Input: dimensioned drawing with shaded views. Units: mm. Origin: part minimum x, y, z. Coordinates: 2 decimals unless noted, no trailing zeros. Order: outer loops, then holes, each group sorted by start corner. A loop starts at its lowest first (then second) coordinate and runs counter-clockwise, first axis right, second up. Notation, with made-up numbers: (-13.75, 37.25) -> (-1.75, 37.25) arc R20 cw to (-1.75, 67.25) -> close; hole circle Ø9 at (-35, 73.5). An arc over 180 degrees is marked (long way). Answer as CSV lines item,"result".
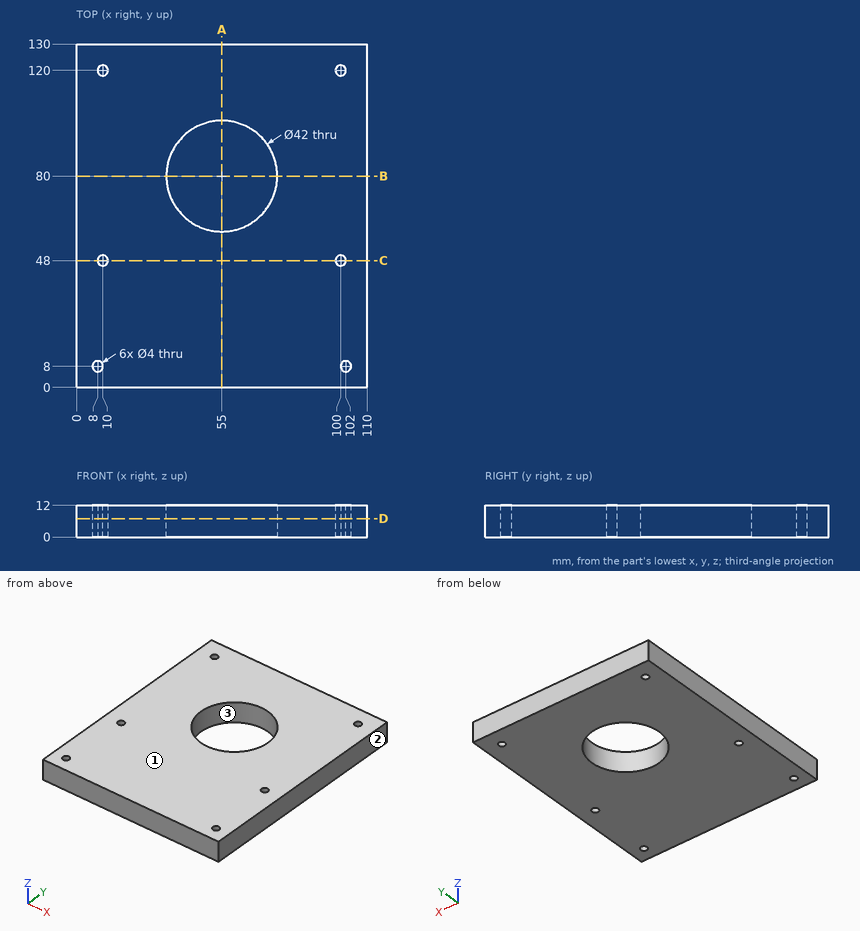
1. Contact query for flat-ended pins moving along their axis: pin 1 (5 mm diameter, centred on y = 20, z = 5.5, fed in from -X); pin 2 (3 mm diameter, centred on x = 102, y = 8, fed in from +Z). Output: stop coordinate, or through.
Findings:
pin 1,"stops at x = 0"
pin 2,"passes through"
2. Cut plane C-C (y = 48). Return the cut outline in (x, z), plus the area to 3 significant figures.
Findings:
outline,"(0, 0) -> (8, 0) -> (8, 12) -> (0, 12) -> close; (12, 0) -> (98, 0) -> (98, 12) -> (12, 12) -> close; (102, 0) -> (110, 0) -> (110, 12) -> (102, 12) -> close"
area,"1,220 mm2"
3. Cut plane A-A (x = 55). Return the cut outline in (y, z), plus the area to 3 significant figures.
Findings:
outline,"(0, 0) -> (59, 0) -> (59, 12) -> (0, 12) -> close; (101, 0) -> (130, 0) -> (130, 12) -> (101, 12) -> close"
area,"1,060 mm2"
4. Cut plane D-D (z = 7). Return the cut outline in (x, y).
Findings:
outline,"(0, 0) -> (110, 0) -> (110, 130) -> (0, 130) -> close; hole circle Ø4 at (8, 8); hole circle Ø4 at (10, 48); hole circle Ø4 at (10, 120); hole circle Ø42 at (55, 80); hole circle Ø4 at (100, 48); hole circle Ø4 at (100, 120); hole circle Ø4 at (102, 8)"
5. Mould query, pull axis X, two halves, no side actions, for the marked faces 1, 2 and 3. Classes: released by +X, released by -X, zero draft, split by the parting line, or undercut.
Findings:
face 1,"zero draft"
face 2,"released by +X"
face 3,"undercut"
6. Cut plane B-B (y = 80). Return the cut outline in (x, z), plus the area to 3 significant figures.
Findings:
outline,"(0, 0) -> (34, 0) -> (34, 12) -> (0, 12) -> close; (76, 0) -> (110, 0) -> (110, 12) -> (76, 12) -> close"
area,"816 mm2"
7. Ray query, line 1 along X through (y, z) = (8, 7.5); line 2 along X through (y, z) = (120, 3); line 3 along Y through (x, z) = (99, 1.5). Return the intervals inside material, ascending.
Findings:
line 1,"x = 0 to 6, 10 to 100, 104 to 110"
line 2,"x = 0 to 8, 12 to 98, 102 to 110"
line 3,"y = 0 to 46.27, 49.73 to 118.27, 121.73 to 130"
